Build history of the part. All positions in model axes, mm. Face numbers are marked on the shaded views. A direction names the side the tool comes from. Give positions to 0.01 mm unless a question says otherwise; leave off trailing zeros. Loops run counter-clockwise (first coordinate to the right, second up) from the corner with the lowest first, then second, coordinate; pieces in that order, holes last. Notation, with made-up numbers: M 79,87.25 L 94,87.25 A14 cw 94,91.25 Z; hole C 2,31 d3. An arc over 180 degrees is marked long. Put each result on its own line as item: value.
```python
from build123d import *

# Parameters (mm, degrees)
F0_W      = 38.1
F0_H      = 38.1
F1_DEPTH  = 38.1
F6_DEPTH  = 38.1
F8_DEPTH  = 38.1
F9_W      = 25.4
F9_H      = 7.62
F9_H_2    = 7.619996
F10_DEPTH = 38.1


with BuildPart() as f1:
    # F0 (on Front) → F1 (new body)
    with BuildSketch(Plane.XZ):
        with Locations((19.05, 19.05)):
            Rectangle(F0_W, F0_H)
    extrude(amount=F1_DEPTH)

    # F5 (on offset) → F6 (cut)
    with BuildSketch(Plane.YZ.offset(38.1)):
        Polygon((-11.43, 14.807015), (-6.35, 38.1), (-31.75, 38.1), (-26.67, 16.386524), (-21.59, 28.575), (-16.51, 28.575), align=None)
        Polygon((-25.4, 0), (-12.7, 0), (-19.05, 15.875), align=None)
        Polygon((-38.1, 0), (-31.75, 0), (-38.1, 38.1), align=None)
        Polygon((-6.35, 0), (0, 0), (0, 38.1), align=None)
    extrude(amount=-F6_DEPTH, mode=Mode.SUBTRACT)

    # F7 (on offset) → F8 (cut)
    with BuildSketch(Plane.XZ.offset(38.1)):
        Polygon((11.43, 22.225), (6.35, 0), (31.75, 0), (26.67, 22.225), (21.59, 9.525), (16.51, 9.525), align=None)
        Polygon((0, 38.1), (0, 0), (6.35, 38.1), align=None)
        Polygon((25.4, 38.1), (12.7, 38.1), (19.05, 22.225), align=None)
        Polygon((31.75, 38.1), (38.100006, 0), (38.100006, 38.1), align=None)
    extrude(amount=-F8_DEPTH, mode=Mode.SUBTRACT)

    # F9 (on offset) → F10 (cut)
    with BuildSketch(Plane.XY.offset(38.1)):
        with Locations((25.4, -11.43)):
            Rectangle(F9_W, F9_H)
        with Locations((12.7, -26.669998)):
            Rectangle(F9_W, F9_H_2)
    extrude(amount=-F10_DEPTH, mode=Mode.SUBTRACT)


solid = f1.part
```
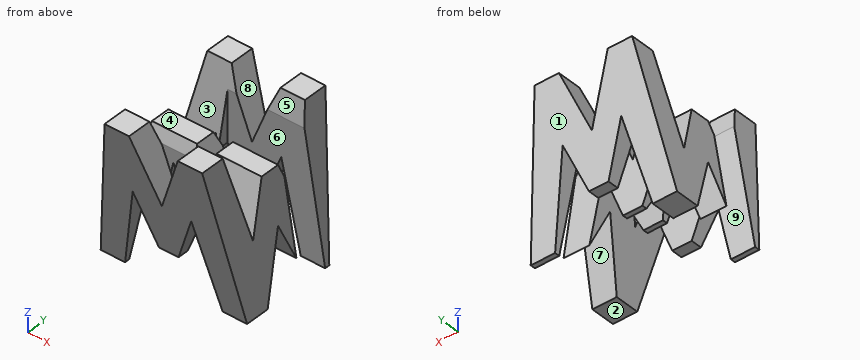
Q1. Slice it at C-C (z = 31.5). List the corners of the cut face in (x, y).
Here are the results:
outline: M 5.25,-37 L 15.34,-37 L 15.34,-30.48 L 5.25,-30.48 Z; M 5.25,-7.79 L 12.7,-7.79 L 12.7,-7.62 L 15.34,-7.62 L 15.34,-1.1 L 5.25,-1.1 Z; M 22.76,-37 L 32.85,-37 L 32.85,-30.21 L 25.4,-30.21 L 25.4,-30.48 L 22.76,-30.48 Z; M 22.76,-7.62 L 32.85,-7.62 L 32.85,-1.1 L 22.76,-1.1 Z
Q2. Drop flat-ended pins along their axis: pin 1 Ø21 at (x, z) = (9.5, 14.5) entering from -Y; pin 2 Ø2.5 at (x, y) = (27, -20) entering from +Z (3 decimals); pin 3 Ø1.3 at (y, z) = (-24, 23) entering from -X; pin 4 Ø1 at (y, z) = (-28.5, 31.5) entering from +X. Give the stop position or say it passes through.
Here are the results:
pin 1: y = -35.92
pin 2: z = 28.575
pin 3: x = 25.4
pin 4: through
Q3. Tool access for the marked faces 5, 6, 7, 8 and 9: list every direction of +Z, -Z, +X, -X, +Y, -Y with a clear straight run to the whole face (end or side of a thin tool).
Here are the results:
face 5: +Z, +X, -X
face 6: +Z, -Z, +X
face 7: -Z, +X, -X
face 8: +Z, +Y, -Y
face 9: +Z, -Z, -X
Q4. Probe line 1 (Y direction, x = 10.5, z = 22.5); line 2 (Y direction, x = 17, z = 12.5); line 3 (Y direction, x = 27.5, z = 25.5). List the from-to ranges inside material, lowest first. Write a range as from..to.
Here are the results:
line 1: -35.5..-30.48, -22.86..-14.27, -9.75..-2.6
line 2: -33.83..-30.48, -22.86..-20.4, -17.7..-15.24, -7.62..-4.27
line 3: -36..-28.8, -22.87..-15.38, -7.62..-2.1
Q5. Slice it at D-D (z = 21). State how many separate pieces and enclosed holes the cut face has, and give its area (3 significant figures).
Here are the results:
separate pieces: 9
enclosed holes: 0
area: 580 mm²
Q6. Slice it at A-A (z = 4). List the corners of the cut face in (x, y).
Here are the results:
outline: M 0.67,-32.42 L 7.26,-32.42 L 7.26,-30.48 L 0.67,-30.48 Z; M 0.67,-14.3 L 7.26,-14.3 L 7.26,-5.68 L 0.67,-5.68 Z; M 30.84,-32.42 L 37.43,-32.42 L 37.43,-23.8 L 30.84,-23.8 Z; M 30.84,-7.62 L 37.43,-7.62 L 37.43,-5.68 L 30.84,-5.68 Z
Q7. Mould opens along Y. For the marked faces 1, 2, 3 and 4 say: pulls with the +Y half, pulls with the -Y half, needs draft (parallel to the pull), parting line crosses it, or undercut.
Here are the results:
face 1: pulls with the +Y half
face 2: needs draft
face 3: undercut
face 4: undercut
